Source: CAD feature listing. Evaluate the final solid. Frame: model axes, mm. Round coordinates to 2 decimals unless told otherwise and drop trailing zeros. Order: outer loops, then holes, each group sorted by start corner. A loop starts at its lowest first (then second) coordinate and runs counter-clockwise, first axis right, second up. Notation, with made-up numbers: (33, -29) -> (89, -29) arc R7 cw to (89, -25) -> close; hole circle Ø5 at (-10.5, -25.5). An arc over 180 degrees is marked (long way). Answer as CSV lines item,"result". Start each with the question number.
(1) Contact query for a flat-ended pin moving along its axis: P1, Ø3, axis at y = -13.71, z = 36.23, coming from the +X side. Output: stop coordinate, or through.
(2) Section query A-A (y = -62.5). Output: boundary loops of the cut face in (x, z).
(3) Line query: line 1 along Z through (x, y) = (0.85, 17); line 2 along Z through (x, y) = (3.95, -14.5); line 3 along Y through (x, z) = (1.35, 18). Output: solid intervals per line, ascending. Write a range as from..to.
(4) Section query B-B (x = 1.2). Count the separate pieces of the cut face and the enclosed holes in it, plus the area to 3 significant figures.
Autodesk Inventor part; units mm, degrees
ref_plane "YZ Plane" through (0, 0, 0) normal (1, 0, 0) x (0, 1, 0)
ref_plane "XZ Plane" through (0, 0, 0) normal (0, 1, 0) x (-1, 0, 0)
ref_plane "XY Plane" through (0, 0, 0) normal (0, 0, 1) x (1, 0, 0)
sketch "Sketch1" plane through (0, 0, 0) normal (1, 0, 0) x (0, 1, 0)
  line L0 (119.0767, 81.9121) -> (-121.9233, 81.9121)
  line L1 (-121.9233, 81.9121) -> (-121.9233, -0.0879)
  line L2 (-121.9233, -0.0879) -> (119.0767, -0.0879)
  line L3 (119.0767, -0.0879) -> (119.0767, 81.9121)
  circle A0 centre (-54.9233, 40.9121) radius 19
  line L4 (-121.9233, 73.9121) -> (-118.9233, 73.9121)
  line L5 (-118.9233, 73.9121) -> (-118.9233, 7.9121)
  line L6 (-118.9233, 7.9121) -> (-121.9233, 7.9121)
  line L7 (-121.9233, 7.9121) -> (-121.9233, 73.9121)
  circle A1 centre (26.2941, 56.2319) radius 2.35
  circle A2 centre (16.2941, 56.2319) radius 2.35
  circle A3 centre (6.2941, 56.2319) radius 2.35
  circle A4 centre (-3.7059, 56.2319) radius 2.35
  circle A5 centre (-13.7059, 56.2319) radius 2.35
  circle A6 centre (26.2941, 46.2319) radius 2.35
  circle A7 centre (16.2941, 46.2319) radius 2.35
  circle A8 centre (6.2941, 46.2319) radius 2.35
  circle A9 centre (-3.7059, 46.2319) radius 2.35
  circle A10 centre (-13.7059, 46.2319) radius 2.35
  circle A11 centre (26.2941, 36.2319) radius 2.35
  circle A12 centre (16.2941, 36.2319) radius 2.35
  circle A13 centre (6.2941, 36.2319) radius 2.35
  circle A14 centre (-3.7059, 36.2319) radius 2.35
  circle A15 centre (-13.7059, 36.2319) radius 2.35
  circle A16 centre (26.2941, 26.2319) radius 2.35
  circle A17 centre (16.2941, 26.2319) radius 2.35
  circle A18 centre (6.2941, 26.2319) radius 2.35
  circle A19 centre (-3.7059, 26.2319) radius 2.35
  circle A20 centre (-13.7059, 26.2319) radius 2.35
  point P0 (0, 0)
  point P1 (0, 0)
  dimension "d0" = 241
  dimension "d1" = 82
  dimension "d2" = 38
  dimension "d3" = 41
  dimension "d4" = 174
  dimension "d5" = 66
  dimension "d6" = 3
  dimension "d7" = 8
  dimension "d21" = 4.7
  dimension "d24" = 10
  dimension "d27" = 10
extrude "Extrusion1" add sketch "Sketch1" along normal blind 5 contours L3 L2 L1 L6 L5 L4 L0
equation "\"d3\" = 0.5 * d1"
equation "\"d7\" = -0.5 * d5 + 0.5 * d1"
properties part number "inner_3Poke"
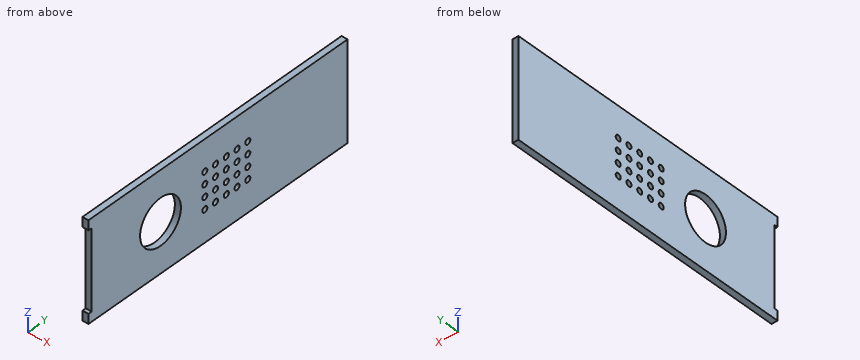
Answer block:
1,P1,"through"
2,outline,"(0, -0.09) -> (5, -0.09) -> (5, 23.49) -> (0, 23.49) -> close; (0, 58.34) -> (5, 58.34) -> (5, 81.91) -> (0, 81.91) -> close"
3,line 1,"-0.09..23.99, 28.47..33.99, 38.47..43.99, 48.47..53.99, 58.47..81.91"
3,line 2,"-0.09..24.02, 28.44..34.02, 38.44..44.02, 48.44..54.02, 58.44..81.91"
3,line 3,"-118.92..119.08"
4,separate pieces,"1"
4,enclosed holes,"21"
4,area,"18,100 mm2"
